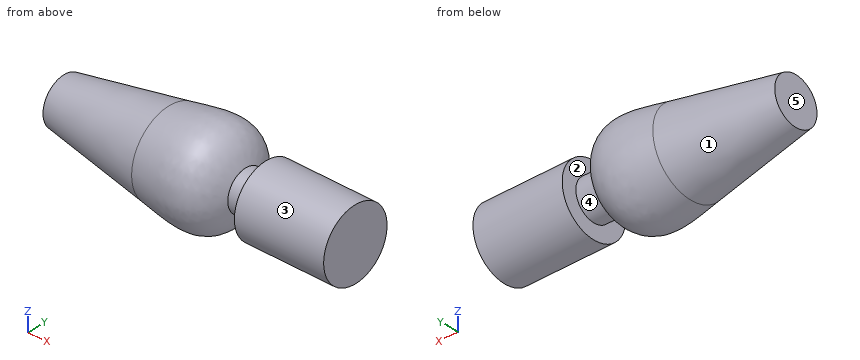
from build123d import *


with BuildPart() as part:
    # Sketch1 → Revolve1 (revolve)
    with BuildSketch(Plane.XY, mode=Mode.PRIVATE) as revolve1_sk:
        with BuildLine():
            Line((6.25, 0), (6.25, 1.5))
            Line((6.25, 1.5), (2.418439441, 1.5))
            Line((2.418439441, 1.5), (2.418439441, 0.85342731))
            Line((2.418439441, 0.85342731), (1.547351676, 0.85342731))
            add(Edge.make_bspline(
                [(-1.732235322, 1.787144344), (-0.144941343, 2.063703564), (0.965721254, 2.439168447), (1.547351676, 0.85342731)],
                knots=[0, 0, 0, 0, 1, 1, 1, 1], degree=3))
            Line((-1.732235322, 1.787144344), (-6.25, 1))
            Line((-6.25, 1), (-6.25, 0))
            Line((-6.25, 0), (6.25, 0))
        make_face()
    revolve(revolve1_sk.sketch.rotate(Axis((-6.25, 0, 0), (1, 0, 0)), 180), axis=Axis((-6.25, 0, 0), (1, 0, 0)))


solid = part.part
The listing builds one solid part. Answer for the finished solid, in the listing's coordinates (mm). Face numbers are marked on the shaded views. A direction names the side the tool comes from. Give positions to 0.01 mm unless a question says otherwise; leave off trailing zeros. Write each loop counter-clockwise with the first axis right and the second up, starting at its lowest first coordinate (ties: lowest second). Pieces come first, ordered by that corner, then holes.
1) A tool of negligible diameter and unlimited length cuts with its end or side. For the marked faces 1 and 2, from which of +Z, -Z, +X, -X, +Y, -Y can it reach the whole face along a straight path? Write none if from no direction.
2) Section A-A (x = 4.25) is taken. Write down the section's boundary in (y, z), and give its area (3 significant figures).
3) For a pull along X with two mould halves and no side action, classify the marked faces 3, 4 and 5 as pulls with the +X half, pulls with the -X half, needs draft (parallel to the pull), parting line crosses it, or undercut.
4) Find the intervals of material crossed by L1, parallel to Y at x = -1, z = -1.1; L2, parallel to Z at x = 0, y = -1.6; L3, parallel to Y at x = 2.75, z = 0.6, in increasing order.
5) Given P1, Ø1, axis at x = -4, y = -1, coming from the -Z side; P2, Ø2, axis at x = -3, z = 0.5, coming from the -Y side, each flat-ended and moving along its own axis, determine where each tip first touches the part or whether it passes through.
Response:
1. face 1: -X
1. face 2: none
2. outline: circle Ø3 at (0, 0)
2. area: 7.07 mm2
3. face 3: needs draft
3. face 4: undercut
3. face 5: pulls with the -X half
4. L1: y = -1.57 to 1.57
4. L2: z = -1.26 to 1.26
4. L3: y = -1.37 to 1.37
5. P1: stops at z = -1.32
5. P2: stops at y = -1.72
